The listing builds one solid part. Answer for the finished solid, in the listing's coordinates (mm). Round coordinates to 2 decimals unless told otherwise and drop trailing zeros. Loops run counter-clockwise (first coordinate to the right, second up) from the corner with the lowest first, then second, coordinate; pieces in that order, holes last. Notation, with made-up numbers: (31.5, -4.5) - (44.5, -4.5) arc R23 cw to (44.5, 9.5) - close; hole circle Ø9 at (77.25, -7). An arc over 180 degrees is marked (long way). One line per question, with ' | ' between items. Start each with the question number.
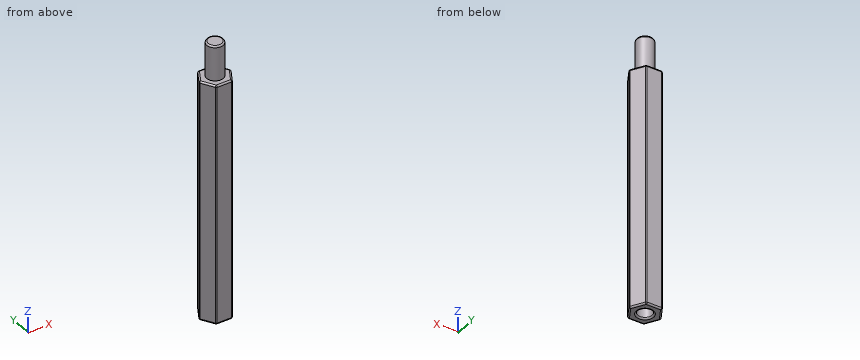
Autodesk Inventor part; units mm, degrees
ref_plane "YZ Plane" through (0, 0, 0) normal (1, 0, 0) x (0, 1, 0)
ref_plane "XZ Plane" through (0, 0, 0) normal (0, 1, 0) x (-1, 0, 0)
ref_plane "XY Plane" through (0, 0, 0) normal (0, 0, 1) x (1, 0, 0)
sketch "Boceto1" plane through (0, 0, 0) normal (0, 0, 1) x (1, 0, 0)
  line L0 (1.3423, 2.325) -> (2.6847, 0)
  line L1 (2.6847, 0) -> (1.3423, -2.325)
  line L2 (1.3423, -2.325) -> (-1.3423, -2.325)
  line L3 (-1.3423, -2.325) -> (-2.6847, 0)
  line L4 (-2.6847, 0) -> (-1.3423, 2.325)
  line L5 (-1.3423, 2.325) -> (1.3423, 2.325)
  point P0 (0, 0)
  point P1 (0, 0)
  point P2 (0, 0)
  dimension "d0" = 4.65
extrude "Extrusión1" add sketch "Boceto1" along normal blind 40
sketch "Boceto2" plane through (0, 0, 40) normal (0, 0, 1) x (1, 0, 0)
  circle A0 centre (0, 0) radius 1.375
  dimension "d3" = 2.75
extrude "Extrusión2" add sketch "Boceto2" along normal blind 5.8
fillet "Empalme1" radius 0.25 1 edges at (-1.375, 0, 45.8)
fillet "Empalme2" radius 0.25 18 edges at (-1.3423, 2.325, 20) (-2.6847, 0, 20) (1.3423, 2.325, 20) (2.6847, 0, 20) (1.3423, -2.325, 20) (-1.3423, -2.325, 20) (0, -2.325, 0) (-2.0135, -1.1625, 0) (-2.0135, 1.1625, 0) (2.0135, 1.1625, 0) (2.0135, -1.1625, 0) (0, 2.325, 0) (2.0135, -1.1625, 40) (0, -2.325, 40) (-2.0135, -1.1625, 40) (-2.0135, 1.1625, 40) (0, 2.325, 40) (2.0135, 1.1625, 40)
sketch "Boceto3" plane through (0, 0, 0) normal (0, 0, -1) x (-1, 0, 0)
  circle A0 centre (0, 0) radius 1.2
  dimension "d8" = 2.4
extrude "Extrusión3" cut sketch "Boceto3" against normal blind 4
fillet "Empalme3" radius 0.25 1 edges at (1.2, 0, 0)
properties part number "Espaciador_40mm"
(1) Find section A-A on x = 0. Write down the section's boundary in (y, z) (3 decimals).
(2) Each of these flat-tipped pins is pushed along its axis until it touches: P1, Ø1.5, axis at y = -1, z = 30.5, coming from the +X side; P2, Ø1.5, axis at x = 1, y = 1.5, coming from the -Z side; P3, Ø1.5, axis at y = -1.5, z = 37, coming from the -X side. Where does it stop, or does it pass through?
(3) Find section B-B on z = 9. Write down the section's boundary in (x, y) (3 decimals).
(4) Consider L1, parallel to Y at x = 0, z = 1.15 (3 decimals); L2, parallel to Z at x = -0.15, y = 1.5; L3, parallel to Z at x = 0.85, y = 0.75. Determine where each line is inside the solid, lowest interval first.
Answer below:
1) outline: (-2.325, 0.25) arc R0.25 ccw to (-2.075, 0) - (-1.45, 0) arc R0.25 ccw to (-1.2, 0.25) - (-1.2, 4) - (1.2, 4) - (1.2, 0.25) arc R0.25 ccw to (1.45, 0) - (2.075, 0) arc R0.25 ccw to (2.325, 0.25) - (2.325, 39.75) arc R0.25 ccw to (2.075, 40) - (1.375, 40) - (1.375, 45.55) arc R0.25 ccw to (1.125, 45.8) - (-1.125, 45.8) arc R0.25 ccw to (-1.375, 45.55) - (-1.375, 40) - (-2.075, 40) arc R0.25 ccw to (-2.325, 39.75) - close
2) P1: x = 2.54 | P2: z = 0 | P3: x = -2.25
3) outline: (-2.613, -0.125) - (-1.414, -2.2) arc R0.25 ccw to (-1.198, -2.325) - (1.198, -2.325) arc R0.25 ccw to (1.414, -2.2) - (2.613, -0.125) arc R0.25 ccw to (2.613, 0.125) - (1.414, 2.2) arc R0.25 ccw to (1.198, 2.325) - (-1.198, 2.325) arc R0.25 ccw to (-1.414, 2.2) - (-2.613, 0.125) arc R0.25 ccw to start
4) L1: -2.325 to -1.2, 1.2 to 2.325 | L2: 0 to 40 | L3: 4 to 45.8
